```python
from build123d import *

# Parameters (mm, degrees)
F0_R     = 4.445
F0_R_2   = 3.175
F0_R_3   = 12.7
F0_R_4   = 5.08
F1_DEPTH = 6.35


with BuildPart() as f1:
    # F0 (on Top) → F1 (new body)
    with BuildSketch(Plane.XY):
        with BuildLine():
            Line((-38.1, -38.1), (38.1, -38.1))
            ThreePointArc((38.1, -38.1), (91.981537, 91.981537), (-38.1, 38.1))
            Line((-38.1, 38.1), (-38.1, -38.1))
        make_face()
        with Locations((16.102955, 25.4)):
            Circle(F0_R, mode=Mode.SUBTRACT)
        with Locations((60.097045, 25.4)):
            Circle(F0_R_2, mode=Mode.SUBTRACT)
        with Locations((38.1, 38.1)):
            Circle(F0_R_3, mode=Mode.SUBTRACT)
        with Locations((38.1, 63.5)):
            Circle(F0_R_4, mode=Mode.SUBTRACT)
    extrude(amount=F1_DEPTH)


solid = f1.part
```
Here's how the part is built. I have some questions about the finished solid (model axes, mm). Coordinates: 2 decimals unless noted, no trailing zeros. Order: outer loops, then holes, each group sorted by start corner. A loop starts at its lowest first (then second) coordinate and runs counter-clockwise, first axis right, second up. Notation, with made-up numbers: M 74,43.25 L 132,43.25 A19 cw 132,79.25 Z; hole C 80.25,-2 d2. An arc over 180 degrees is marked long. Answer as a JSON object with one key per item and string values. Group by question number.
(1) I need wall thicknesses on probe 1 along Y at (x, z) = (38.1, 5); probe 2 along X at (y, z) = (37, 3); probe 3 along Y at (x, z) = (23.5, 3.75). Which ranges of each line are inside material? Lowest first, please.
(2) Suppose I cut it at D-D, the plane y = 79.5. Please give me the cut outline in (x, z), then the cut area to 3 significant figures.
(3) For pin 1 (15 mm diameter, centred on x = 38.1, y = 38.1, fed in from -Z); pin 2 (2 mm diameter, centred on y = 1.5, z = 3, fed in from +X); pin 3 (3 mm diameter, centred on y = -4, z = 1.5, fed in from +X); pin 4 (3 mm diameter, centred on y = 39, z = 2.5, fed in from +X), each with a flat end and sliding along its axis, tell me the tip position at first contact or that it passes through.
(4) Suppose I cut it at A-A, the plane z = 3.25. Please give me the cut outline in (x, y) (3 decimals).
(5) If we mould it in two halves opening along Y, with no side actions, what happens to faces 1 (the face through (37, 22, 6.35)), 2 (the face through (-1, -38.1, 3)), 3 (the face through (20.21, 23.7, 3.13)), 4 (the face through (93.729, 90.175, 3.131))? For each: released by +Y, released by -Y, zero draft, split by the parting line, or undercut.
(6) Suppose I cut it at B-B, the plane y = 63.5. Please give me the cut outline in (x, z).
(7) Suppose I cut it at C-C, the plane x = 40.5. Please give me the cut outline in (y, z).
Values found:
{
 "1": {"probe 1": "y = -38.1 to 25.4, 50.8 to 58.42, 68.58 to 114.3", "probe 2": "x = -38.1 to 25.45, 50.75 to 114.29", "probe 3": "y = -38.1 to 112.89"},
 "2": {"outline": "M -25.87,0 L 102.07,0 L 102.07,6.35 L -25.87,6.35 Z", "area": "812 mm^2"},
 "3": {"pin 1": "passes through", "pin 2": "stops at x = 105.47", "pin 3": "stops at x = 102.58", "pin 4": "stops at x = 114.3"},
 "4": {"outline": "M -38.1,-38.1 L 38.1,-38.1 A76.2 ccw long -38.1,38.1 Z; hole C 16.103,25.4 d8.89; hole C 38.1,38.1 d25.4; hole C 38.1,63.5 d10.16; hole C 60.097,25.4 d6.35"},
 "5": {"face 1": "zero draft", "face 2": "released by -Y", "face 3": "undercut", "face 4": "split by the parting line"},
 "6": {"outline": "M -33.74,0 L 33.02,0 L 33.02,6.35 L -33.74,6.35 Z; M 43.18,0 L 109.94,0 L 109.94,6.35 L 43.18,6.35 Z"},
 "7": {"outline": "M -38.06,0 L 25.63,0 L 25.63,6.35 L -38.06,6.35 Z; M 50.57,0 L 59.02,0 L 59.02,6.35 L 50.57,6.35 Z; M 67.98,0 L 114.26,0 L 114.26,6.35 L 67.98,6.35 Z"}
}
